For this review, take the finished solid that the model builds, in its own axes (mm). A direction names the side the tool comes from. Coordinates: 2 decimals unless noted, no trailing zeros. Write each loop counter-clockwise with the first axis right and the second up, starting at its lowest first coordinate (ties: lowest second). Pieces come first, ordered by that corner, then holes. Notation, with made-up numbers: M 74,4.5 L 97,4.5 A13 ccw 97,16.5 Z; hole C 48,13 d8. An arc over 180 degrees is marked long. One line per question, with ' | ' between items.
from build123d import *

# Parameters (mm, degrees)
BOSS_EXTRUDE1_REACH = 9
SKETCH2_R           = 3.96875


with BuildPart() as part:
    # Sketch1 → Revolve1 (revolve)
    with BuildSketch(Plane(origin=(0, 0, 0), x_dir=(0, 0, -1), z_dir=(1, 0, 0))):
        Polygon((0, 3.96875), (-7, 3.96875), (-7, 4.7625), (-3.625, 4.7625), (-1.5875, 6.8), (0, 6.8), align=None)
    revolve(axis=Axis((0, 0, 0), (0, 0, 1)))

    # Sketch2 → Boss-Extrude1 (add, up to next)
    with BuildSketch(Plane.XY.offset(7), mode=Mode.PRIVATE) as boss_extrude1_sk1:
        Polygon((-2.886751346, 5), (-5.773502692, 0), (-2.886751346, -5), (2.886751346, -5), (5.773502692, 0), (2.886751346, 5), align=None)
        Circle(SKETCH2_R, mode=Mode.SUBTRACT)
    boss_extrude1_tool1 = extrude(boss_extrude1_sk1.sketch, amount=-BOSS_EXTRUDE1_REACH, mode=Mode.PRIVATE) - part.part
    add(boss_extrude1_tool1.solids().sort_by_distance((-4.197839, 2.423624, 7))[0])


solid = part.part
1. Draft analysis for pull direction Y (two halves, no side actions). For faces 4 (the flat face through (3, 3, 0)), 5 (the cylindrical face through (3.874, -0.86, 3.549)), 6 (the flat face through (0, -5, 5)), state which applies: pulls with the +Y half, pulls with the -Y half, needs draft (parallel to the pull), parting line crosses it, or undercut.
Computed values:
face 4: needs draft | face 5: undercut | face 6: pulls with the -Y half
2. Take a section at A-A on z = 6. State the section outline as (x, y) points.
Computed values:
outline: M -5.77,0 L -2.89,-5 L 2.89,-5 L 5.77,0 L 2.89,5 L -2.89,5 Z; hole C 0,0 d7.94
3. Clearance check with flat-ended pins moving along their axes: P1, Ø1.3, axis at x = 0.5, z = 5, coming from the -Y side; P2, Ø3, axis at y = 3.5, z = 1.5, coming from the +X side; P3, Ø4, axis at x = 2.5, z = 2.5, coming from the -Y side. State where each tip first meets the part, or that it passes through.
Computed values:
P1: stops at y = -5 | P2: stops at x = 6.5 | P3: stops at y = -6.76
4. Machinability: for faces 1 (the flat face through (-4.35, -2.465, 4.838)), 2 (the flat face through (4.35, 2.465, 4.838)), 3 (the flat face through (4.31, -2.535, 4.838)), which of the approach directions +Z, -Z, +X, -X, +Y, -Y give a long, thin tool a straight path to every point of the face, cutting with its end or side? Answer none if there is none.
Computed values:
face 1: +Z, -X, -Y | face 2: +Z, +X, +Y | face 3: +Z, +X, -Y
5. Take a section at C-C on z = 0.5. State the section outline as (x, y) points.
Computed values:
outline: C 0,0 d13.6; hole C 0,0 d7.94
6. For line 1 along Y through (x, z) = (0, 5.75); line 2 along X through (y, z) = (0, 1.5); line 3 along X through (y, z) = (0, 2.25), list the stretches that pass through material, from the lowest coordinate up.
Computed values:
line 1: y = -5 to -3.97, 3.97 to 5 | line 2: x = -6.8 to -3.97, 3.97 to 6.8 | line 3: x = -6.14 to -3.97, 3.97 to 6.14
7. Take a section at B-B on x = 0. State the section outline as (y, z) points.
Computed values:
outline: M -6.8,0 L -3.97,0 L -3.97,7 L -5,7 L -5,3.39 L -6.8,1.59 Z; M 3.97,0 L 6.8,0 L 6.8,1.59 L 5,3.39 L 5,7 L 3.97,7 Z
